```python
from build123d import *

# Parameters (mm, degrees)
SKETCH_1_R          = 47.75
EXTRUDE_1_DEPTH     = 3
CUT_EXTRUDE_1_DEPTH = 68.595303091
SKETCH_3_R          = 1.525
CUT_EXTRUDE_2_DEPTH = 68.564300519
SKETCH_4_R          = 27.5
CUT_EXTRUDE_3_DEPTH = 68.564300519
FILLET_1_R          = 2


with BuildPart() as part:
    # ｽｹｯﾁ1 → ﾎﾞｽ - 押し出し1 (new body)
    with BuildSketch(Plane.XY):
        Circle(SKETCH_1_R)
    extrude(amount=EXTRUDE_1_DEPTH)

    # ｽｹｯﾁ2 → ｶｯﾄ - 押し出し1 (cut, through all)
    with BuildSketch(Plane.XY.offset(3)):
        with BuildLine():
            Line((-10.3, 46.625878008), (-10.3, 32.325692416))
            ThreePointArc((-10.3, 32.325692416), (0, 31.28), (10.3, 32.325692416))
            Line((10.3, 32.325692416), (10.3, 46.625878008))
            ThreePointArc((10.3, 46.625878008), (0, 47.75), (-10.3, 46.625878008))
        make_face()
        with BuildLine():
            Line((22.08027891, 42.338207133), (12.888296795, 31.383629425))
            ThreePointArc((12.888296795, 31.383629425), (20.106396431, 23.961870181), (28.668812324, 18.142204665))
            Line((28.668812324, 18.142204665), (37.860794438, 29.096782374))
            ThreePointArc((37.860794438, 29.096782374), (30.693108363, 36.578622159), (22.08027891, 42.338207133))
        make_face()
        with BuildLine():
            Line((44.128949923, 18.240018604), (30.046016283, 15.756817436))
            ThreePointArc((30.046016283, 15.756817436), (30.804786514, 5.431714997), (33.623168743, -4.530222276))
            Line((33.623168743, -4.530222276), (47.706102383, -2.047021108))
            ThreePointArc((47.706102383, -2.047021108), (47.024570206, 8.291700484), (44.128949923, 18.240018604))
        make_face()
        with BuildLine():
            Line((45.529194829, -14.392877345), (33.144870827, -7.242784549))
            ThreePointArc((33.144870827, -7.242784549), (27.08927463, -15.64), (22.844870827, -25.082907867))
            Line((22.844870827, -25.082907867), (35.229194829, -32.233000663))
            ThreePointArc((35.229194829, -32.233000663), (41.352713031, -23.875), (45.529194829, -14.392877345))
        make_face()
        with BuildLine():
            Line((25.625823473, -40.291186025), (20.734871947, -26.853407149))
            ThreePointArc((20.734871947, -26.853407149), (10.698390083, -29.393585178), (1.377203959, -33.899022101))
            Line((1.377203959, -33.899022101), (6.268155485, -47.336800978))
            ThreePointArc((6.268155485, -47.336800978), (16.331461844, -44.870322643), (25.625823473, -40.291186025))
        make_face()
        with BuildLine():
            Line((-6.268155485, -47.336800978), (-1.377203959, -33.899022101))
            ThreePointArc((-1.377203959, -33.899022101), (-10.698390083, -29.393585178), (-20.734871947, -26.853407149))
            Line((-20.734871947, -26.853407149), (-25.625823473, -40.291186025))
            ThreePointArc((-25.625823473, -40.291186025), (-16.331461844, -44.870322643), (-6.268155485, -47.336800978))
        make_face()
        with BuildLine():
            Line((-35.229194829, -32.233000663), (-22.844870827, -25.082907867))
            ThreePointArc((-22.844870827, -25.082907867), (-27.08927463, -15.64), (-33.144870827, -7.242784549))
            Line((-33.144870827, -7.242784549), (-45.529194829, -14.392877345))
            ThreePointArc((-45.529194829, -14.392877345), (-41.352713031, -23.875), (-35.229194829, -32.233000663))
        make_face()
        with BuildLine():
            Line((-47.706102383, -2.047021108), (-33.623168743, -4.530222276))
            ThreePointArc((-33.623168743, -4.530222276), (-30.804786514, 5.431714997), (-30.046016283, 15.756817436))
            Line((-30.046016283, 15.756817436), (-44.128949923, 18.240018604))
            ThreePointArc((-44.128949923, 18.240018604), (-47.024570206, 8.291700484), (-47.706102383, -2.047021108))
        make_face()
        with BuildLine():
            Line((-37.860794438, 29.096782374), (-28.668812324, 18.142204665))
            ThreePointArc((-28.668812324, 18.142204665), (-20.106396431, 23.961870181), (-12.888296795, 31.383629425))
            Line((-12.888296795, 31.383629425), (-22.08027891, 42.338207133))
            ThreePointArc((-22.08027891, 42.338207133), (-30.693108363, 36.578622159), (-37.860794438, 29.096782374))
        make_face()
    extrude(amount=-CUT_EXTRUDE_1_DEPTH, mode=Mode.SUBTRACT)

    # ｽｹｯﾁ3 → ｶｯﾄ - 押し出し2 (cut, through all)
    with BuildSketch(Plane.XY.offset(3)):
        with Locations((0, -38.5)):
            Circle(SKETCH_3_R)
        with Locations((-24.747322973, -29.49271106)):
            Circle(SKETCH_3_R)
        with Locations((-37.915098491, -6.68545484)):
            Circle(SKETCH_3_R)
        with Locations((-33.341978046, 19.25)):
            Circle(SKETCH_3_R)
        with Locations((-13.167775518, 36.1781659)):
            Circle(SKETCH_3_R)
        with Locations((13.167775518, 36.1781659)):
            Circle(SKETCH_3_R)
        with Locations((33.341978046, 19.25)):
            Circle(SKETCH_3_R)
        with Locations((37.915098491, -6.68545484)):
            Circle(SKETCH_3_R)
        with Locations((24.747322973, -29.49271106)):
            Circle(SKETCH_3_R)
    extrude(amount=-CUT_EXTRUDE_2_DEPTH, mode=Mode.SUBTRACT)

    # ｽｹｯﾁ4 → ｶｯﾄ - 押し出し3 (cut, through all)
    with BuildSketch(Plane(origin=(0, 0, 0), x_dir=(-1, 0, 0), z_dir=(0, 0, -1))):
        Circle(SKETCH_4_R)
    extrude(amount=-CUT_EXTRUDE_3_DEPTH, mode=Mode.SUBTRACT)

    # ﾌｨﾚｯﾄ1
    fillet_1_edges = [part.edges().sort_by_distance(p)[0] for p in [
        (-30.046016283, 15.756817436, 1.5),
        (-33.623168743, -4.530222276, 1.5),
        (-47.706102383, -2.047021108, 1.5),
        (-44.128949923, 18.240018604, 1.5),
        (-12.888296795, 31.383629425, 1.5),
        (-28.668812324, 18.142204665, 1.5),
        (-37.860794438, 29.096782374, 1.5),
        (-22.08027891, 42.338207133, 1.5),
        (-20.734871947, -26.853407149, 1.5),
        (-1.377203959, -33.899022101, 1.5),
        (-6.268155485, -47.336800978, 1.5),
        (-25.625823473, -40.291186025, 1.5),
        (-33.144870827, -7.242784549, 1.5),
        (-22.844870827, -25.082907867, 1.5),
        (-35.229194829, -32.233000663, 1.5),
        (-45.529194829, -14.392877345, 1.5),
        (22.844870827, -25.082907867, 1.5),
        (33.144870827, -7.242784549, 1.5),
        (45.529194829, -14.392877345, 1.5),
        (35.229194829, -32.233000663, 1.5),
        (1.377203959, -33.899022101, 1.5),
        (20.734871947, -26.853407149, 1.5),
        (25.625823473, -40.291186025, 1.5),
        (6.268155485, -47.336800978, 1.5),
        (28.668812324, 18.142204665, 1.5),
        (12.888296795, 31.383629425, 1.5),
        (22.08027891, 42.338207133, 1.5),
        (37.860794438, 29.096782374, 1.5),
        (33.623168743, -4.530222276, 1.5),
        (30.046016283, 15.756817436, 1.5),
        (44.128949923, 18.240018604, 1.5),
        (47.706102383, -2.047021108, 1.5),
        (10.3, 32.325692416, 1.5),
        (-10.3, 32.325692416, 1.5),
        (-10.3, 46.625878008, 1.5),
        (10.3, 46.625878008, 1.5),
    ]]
    fillet(fillet_1_edges, radius=FILLET_1_R)


solid = part.part
```
Part model, mm, in its own coordinate system. A direction names the side the tool comes from. Round coordinates to 2 decimals unless told otherwise and drop trailing zeros. Write each loop counter-clockwise with the first axis right and the second up, starting at its lowest first coordinate (ties: lowest second). Pieces come first, ordered by that corner, then holes.
Item 1: Cut at A-A, the plane x = 0. Give the cut face in (y, z) (3 decimals), plus the area to 3 significant figures.
Results:
outline: (-47.75, 0) - (-40.025, 0) - (-40.025, 3) - (-47.75, 3) - close; (-36.975, 0) - (-27.5, 0) - (-27.5, 3) - (-36.975, 3) - close; (27.5, 0) - (31.28, 0) - (31.28, 3) - (27.5, 3) - close
area: 62.9 mm2
Item 2: Cut at D-D, the plane z = 0.6. Count the separate pieces of the cut face and the enclosed holes in it, plus the area to 3 significant figures.
Results:
separate pieces: 1
enclosed holes: 10
area: 1,780 mm2
Item 3: Probe L1, parallel to X at y = -36, z = 2.25; L2, parallel to Y at x = 34.5, z = 0.25; L3, parallel to X at y = -8.5, z = 1.55. List the from-to ranges inside material, lowest first.
Results:
L1: x = -31.37 to -24.06, -2.14 to 2.14, 24.06 to 31.37
L2: y = -8.03 to -4.23, 16.54 to 18.26, 20.24 to 25.09
L3: x = -46.99 to -35.32, -32.07 to -26.15, 26.15 to 32.07, 35.32 to 46.99
Item 4: Cut at C-C, the plane y = 8. Give the cut face in (x, z), plus the area to 3 significant figures.
Results:
outline: (-30.42, 0) - (-26.31, 0) - (-26.31, 3) - (-30.42, 3) - close; (26.31, 0) - (30.42, 0) - (30.42, 3) - (26.31, 3) - close
area: 24.6 mm2
Item 5: Which spindle directions (+Z, -Z, +X, -X, +Y, -Y) get a long thin tool onto all of the face, cutting with end or side? Do faces 1 (the flat face through (-10.3, 39, 2)), 2 (the cylindrical face through (-0.05, -47.75, 1.48)), 3 (the flat face through (-40.29, -3.355, 1.521)), 4 (the flat face through (-36.574, 16.908, 1.521)). Say none if no direction does.
Results:
face 1: +Z, -Z, +Y
face 2: +Z, -Z, -Y
face 3: +Z, -Z
face 4: +Z, -Z, -X
Item 6: Drop flat-ended pins along their axis: pin 1 Ø1.8 at (x, y) = (-24.75, -29.49) entering from +Z; pin 2 Ø0.9 at (y, z) = (38.5, 1.5) entering from +X. Give the stop position or say it passes through.
Results:
pin 1: passes through
pin 2: stops at x = 19.24
Item 7: Cut at B-B, the plane y = 24.5. Give the cut face in (x, z), plus the area to 3 significant figures.
Results:
outline: (-40.99, 0) - (-34, 0) - (-34, 3) - (-40.99, 3) - close; (-19.48, 0) - (-12.49, 0) - (-12.49, 3) - (-19.48, 3) - close; (12.49, 0) - (19.48, 0) - (19.48, 3) - (12.49, 3) - close; (34, 0) - (40.99, 0) - (40.99, 3) - (34, 3) - close
area: 83.8 mm2
Item 8: Two-plate mould, pull along X, no slides. Class faces 5 (the cylindrical face through (-5.18, -46.72, 1.48)), 6 (the cylindrical face through (33.9, -4, 1.5)), 7 (the cylindrical face through (33.993, -32.409, 1.479)): +X half, -X half, draft (parallel to the pull), parting line (faces both ways), or undercut.
Results:
face 5: -X half
face 6: undercut
face 7: +X half
